Work out the finished part from the listing and answer in its coordinate system (mm). Face numbers are marked on the shaded views. A direction names the side the tool comes from. Round coordinates to 2 decimals unless told otherwise and drop trailing zeros. Write each loop counter-clockwise with the first axis right and the second up, starting at its lowest first coordinate (ties: lowest second). Pieces come first, ordered by that corner, then holes. Notation, with made-up numbers: (-24.5, 54.25) -> (22.5, 54.25) arc R21 cw to (22.5, 83.25) -> close; hole circle Ø8 at (45.25, -5). An arc over 180 degrees is marked (long way). One line per item, written item: value.
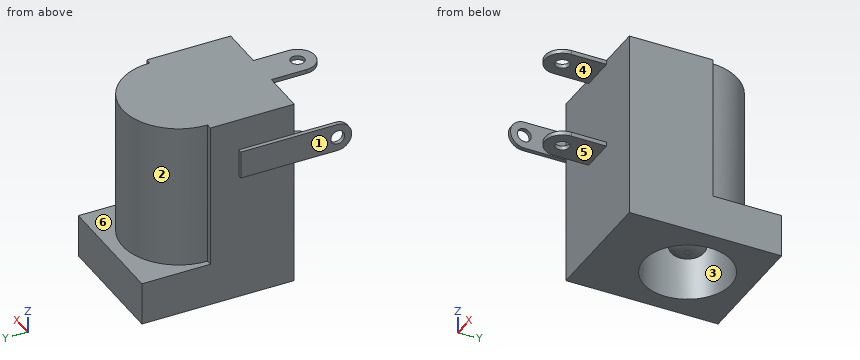
```python
from build123d import *

# Parameters (mm, degrees)
ESBO_O1_W                = 8.9
ESBO_O1_H                = 11
RESSALTO_EXTRUS_O1_DEPTH = 13.6
CORTE_EXTRUS_O1_DEPTH    = 10.5
ESBO_O3_R                = 3.15
CORTE_EXTRUS_O2_DEPTH    = 9.5
ESBO_O4_R                = 1.25
RESSALTO_EXTRUS_O2_DEPTH = 8
FILETE1_SIZE             = 0.5
FILETE1_SIZE_2           = 1
ESBO_O5_W                = 2.5
ESBO_O5_H                = 0.3
RESSALTO_EXTRUS_O3_DEPTH = 3.8
CORTE_EXTRUS_O3_DEPTH    = 10
ESBO_O8_R                = 0.5
CORTE_EXTRUS_O4_DEPTH    = 10
RESSALTO_EXTRUS_O4_DEPTH = 0.3
ESBO_O10_R               = 0.5
CORTE_EXTRUS_O5_DEPTH    = 0.3


with BuildPart() as part:
    # Esboço1 → Ressalto-extrusão1 (new body)
    with BuildSketch(Plane.XY):
        Rectangle(ESBO_O1_W, ESBO_O1_H)
    extrude(amount=RESSALTO_EXTRUS_O1_DEPTH)

    # Esboço2 → Corte-extrusão1 (cut)
    with BuildSketch(Plane.XY.offset(13.6)):
        with BuildLine():
            Line((-4.45, 0.55), (-4.45, 5.5))
            Line((-4.45, 5.5), (4.45, 5.5))
            Line((4.45, 5.5), (4.45, 0.55))
            Line((4.45, 0.55), (4.05, 0.55))
            ThreePointArc((4.05, 0.55), (0, 4.6), (-4.05, 0.55))
            Line((-4.05, 0.55), (-4.45, 0.55))
        make_face()
    extrude(amount=-CORTE_EXTRUS_O1_DEPTH, mode=Mode.SUBTRACT)

    # Esboço3 → Corte-extrusão2 (cut)
    with BuildSketch(Plane(origin=(0, 0, 0), x_dir=(-1, 0, 0), z_dir=(0, 0, -1))):
        with Locations((0, 1)):
            Circle(ESBO_O3_R)
    extrude(amount=-CORTE_EXTRUS_O2_DEPTH, mode=Mode.SUBTRACT)

    # Esboço4 → Ressalto-extrusão2 (add)
    with BuildSketch(Plane(origin=(0, 0, 9.5), x_dir=(-1, 0, 0), z_dir=(0, 0, -1))):
        with Locations((0, 1)):
            Circle(ESBO_O4_R)
    extrude(amount=RESSALTO_EXTRUS_O2_DEPTH)

    # Filete1
    # an asymmetric fillet: 1, 0.5 mm, written as the material it takes off along each edge
    with BuildSketch(Plane(origin=(0, 1, 1.5), x_dir=(-1, 0, 0), z_dir=(0, -1, 0))) as filete1_piece_1:
        with BuildLine():
            Bezier((1.25, -FILETE1_SIZE), (1.25, 0), (1.25 - FILETE1_SIZE_2, 0), weights=[1, 0.707106781, 1])
            Line((1.25 - FILETE1_SIZE_2, 0), (1.25, 0))
            Line((1.25, 0), (1.25, -FILETE1_SIZE))
        make_face()
    revolve(axis=Axis((0, 1, 1.5), (0, 0, -1)), mode=Mode.SUBTRACT)

    # Esboço5 → Ressalto-extrusão3 (add)
    with BuildSketch(Plane.XZ.offset(5.5)):
        with Locations((0, 13.45)):
            Rectangle(ESBO_O5_W, ESBO_O5_H)
        with Locations((0, 7.15)):
            Rectangle(ESBO_O5_W, ESBO_O5_H)
    extrude(amount=RESSALTO_EXTRUS_O3_DEPTH)

    # Esboço7 → Corte-extrusão3 (cut)
    with BuildSketch(Plane.XY.offset(13.6)):
        with BuildLine():
            Line((-1.25, -8.04), (-1.25, -9.3))
            Line((-1.25, -9.3), (1.25, -9.3))
            Line((1.25, -9.3), (1.25, -8.04))
            ThreePointArc((1.25, -8.04), (0, -9.29), (-1.25, -8.04))
        make_face()
    extrude(amount=-CORTE_EXTRUS_O3_DEPTH, mode=Mode.SUBTRACT)

    # Esboço8 → Corte-extrusão4 (cut)
    with BuildSketch(Plane.XY.offset(13.6)):
        with Locations((0, -8.04)):
            Circle(ESBO_O8_R)
    extrude(amount=-CORTE_EXTRUS_O4_DEPTH, mode=Mode.SUBTRACT)

    # Esboço9 → Ressalto-extrusão4 (add)
    with BuildSketch(Plane.ZY.offset(4.45)):
        with BuildLine():
            Line((9.3, -1.5), (11.3, -1.5))
            Line((11.3, -1.5), (11.3, -8.5))
            ThreePointArc((11.3, -8.5), (10.3, -9.5), (9.3, -8.5))
            Line((9.3, -8.5), (9.3, -1.5))
        make_face()
    extrude(amount=RESSALTO_EXTRUS_O4_DEPTH)

    # Esboço10 → Corte-extrusão5 (cut)
    with BuildSketch(Plane.ZY.offset(4.75)):
        with Locations(Location((10.3, -8.5, 0), (0, 0, 270))):
            Circle(ESBO_O10_R)
    extrude(amount=-CORTE_EXTRUS_O5_DEPTH, mode=Mode.SUBTRACT)


solid = part.part
```
(1) Find section A-A on z = 5.25. Give the vertices of the cut face in (x, y), plus the area to 3 significant figures.
Reported:
outline: (-4.45, -5.5) -> (4.45, -5.5) -> (4.45, 0.55) -> (4.05, 0.55) arc R4.05 ccw to (-4.05, 0.55) -> (-4.45, 0.55) -> close; circle Ø2.5 at (0, 1); hole circle Ø6.3 at (0, 1)
area: 53.3 mm2
(2) Find section D-D on x = 0. Give the number of separate pieces and of enclosed holes in the cut face, plus the area to 3 significant figures.
Reported:
separate pieces: 3
enclosed holes: 0
area: 102 mm2
(3) Flat-ended cylindrical pins translate along their axes: pin 1 Ø2.5 at (x, z) = (0.5, 7.5) entering from -Y; pin 2 Ø1 at (x, y) = (-2.5, -1.5) entering from -Z; pin 3 Ø2 at (x, z) = (0, 10.5) entering from +Y; pin 4 Ø0.8 at (x, y) = (0.5, -6.5) entering from -Z. Find the tip coordinate at first contact, or state that the pin passes through.
Reported:
pin 1: stops at y = -9.29
pin 2: stops at z = 0
pin 3: stops at y = 4.6
pin 4: stops at z = 7
(4) Find section C-C on z = 10.3. Give the vertices of the cut face in (x, y), plus the area to 3 significant figures.
Reported:
outline: (-4.75, -9.5) -> (-4.45, -9.5) -> (-4.45, -9) -> (-4.75, -9) -> close; (-4.75, -8) -> (-4.45, -8) -> (-4.45, -5.5) -> (4.45, -5.5) -> (4.45, 0.55) -> (4.05, 0.55) arc R4.05 ccw to (-4.05, 0.55) -> (-4.45, 0.55) -> (-4.45, -1.5) -> (-4.75, -1.5) -> close
area: 81.7 mm2
(5) A tool of negligible diameter and unlimited length cuts with its end or side. For the marked faces 4, 5 and 6, from which of +Z, -Z, +X, -X, +Y, -Y can it reach the whole face along a straight path? Write none if from no direction.
Reported:
face 4: +X, -X, -Y
face 5: -Z, +X, -X, -Y
face 6: +Z, +Y
(6) Find section B-B on y = -6. Give the vertices of the cut face in (x, z).
Reported:
outline: (-4.75, 9.3) -> (-4.45, 9.3) -> (-4.45, 11.3) -> (-4.75, 11.3) -> close; (-1.25, 7) -> (1.25, 7) -> (1.25, 7.3) -> (-1.25, 7.3) -> close; (-1.25, 13.3) -> (1.25, 13.3) -> (1.25, 13.6) -> (-1.25, 13.6) -> close
(7) For a pull along Y with two mould halves and no side action, classify the marked faces 1, 2 and 3 as pulls with the +Y half, pulls with the -Y half, needs draft (parallel to the pull), parting line crosses it, or undercut.
Reported:
face 1: needs draft
face 2: pulls with the +Y half
face 3: undercut
(8) Consider probe 1 along Z at (x, y) = (-4.55, -8.5); probe 2 along Y at (x, z) = (0, 13.5); probe 3 along Z at (x, y) = (-0.5, 4.75). Determine where each line is inside the solid, lowest interval first.
Reported:
probe 1: z = 9.3 to 9.8, 10.8 to 11.3
probe 2: y = -9.29 to -8.54, -7.54 to 4.6
probe 3: z = 0 to 3.1
